Design review of the part shown in the three views and the two pictorial views. Dimensions are in mm from the part's minimum x, y and z. Coordinates: 2 decimals unless noted, no trailing zeros. Loops run counter-clockwise (first coordinate to the right, second up) from the corner with the lowest first, then second, coordinate; pieces in that order, holes last. Notation, with made-up numbers: (33, 74.5) - (80, 74.5) arc R13 ccw to (80, 88.5) - close; hole circle Ø8 at (82.5, 81.25). An arc over 180 degrees is marked (long way). One line per item, written item: value. Start each with the question number.
1. Insertion check: pin 1 (1.9 mm diameter, centred on x = 4, z = 4, fed in from -Y). The pin has a flat end and moves straight along its axis. Give the tip position at first contact, or say it passes through.
2. Take a section at A-A, the plane y = 0.85. State the section outline as (x, z) points.
3. To check wall thickness, follow line 1 (X direction, y = 2, z = 4); line 2 (X direction, y = 2.65, z = 4.5); line 3 (Z direction, x = 137, y = 2.35). State the ranges of each line that lie inside material, in increasing order. Write a range as from..to.
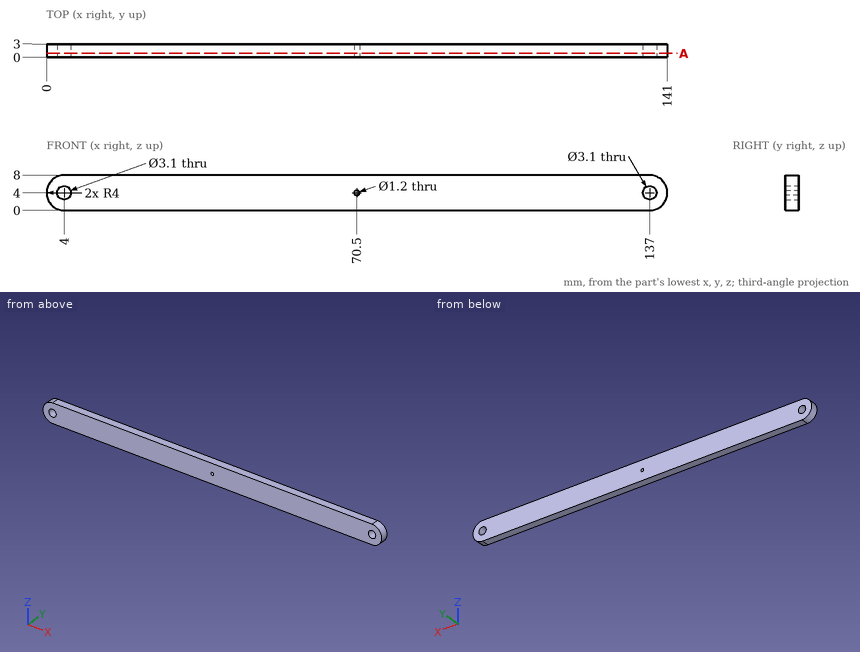
Solutions:
1. pin 1: through
2. outline: (4, 0) - (137, 0) arc R4 ccw to (137, 8) - (4, 8) arc R4 ccw to start; hole circle Ø3.1 at (4, 4); hole circle Ø1.2 at (70.5, 4); hole circle Ø3.1 at (137, 4)
3. line 1: 0..2.45, 5.55..69.9, 71.1..135.45, 138.55..141
3. line 2: 0.03..2.53, 5.47..70.17, 70.83..135.53, 138.47..140.97
3. line 3: 0..2.45, 5.55..8
